Geometry check sheet. Reference: drawing and pictorial views, mm from the part's lowest x, y, z. A direction names the side the tool comes from. Give positions to 0.01 mm unless a question says otherwise; leave off trailing zeros. Write each loop counter-clockwise with the first axis right and the second up, starting at its lowest first coordinate (ties: lowest second). Pieces come first, ordered by that corner, then holes. Notation, with made-up numbers: (64.5, 33.25) - (97.5, 33.25) arc R18 ccw to (97.5, 55.25) - close; hole circle Ø6 at (-9, 28). An arc over 180 degrees is marked (long way). Write item = value, one per line. Start each with the question number.
(1) Section check A-A, the plane x = 3. Enter the section's corners in (y, z), plus the area to 3 significant figures.
(2) Access from +Z, -Z, +X, -X, +Y, -Y to the whole of each face (thin tool, end or side, straight path). Record for the marked faces 1 and 2.
(3) Section check D-D, the plane x = 16.5. Enter the section's corners in (y, z), plus the area to 3 significant figures.
(4) Section check B-B, the plane z = 5.5. Enter the section's corners in (x, y), plus the area to 3 significant figures.
(5) Thickness scan on L1, parallel to Z at x = 6, y = 21; L2, parallel to X at y = 13.5, z = 5; L3, parallel to X at y = 4.75, z = 1.5. Record the ranges inside material, lowest first.
(6) Section check C-C, the plane y = 5. Enter the section's corners in (x, z), plus the area to 3 significant figures.
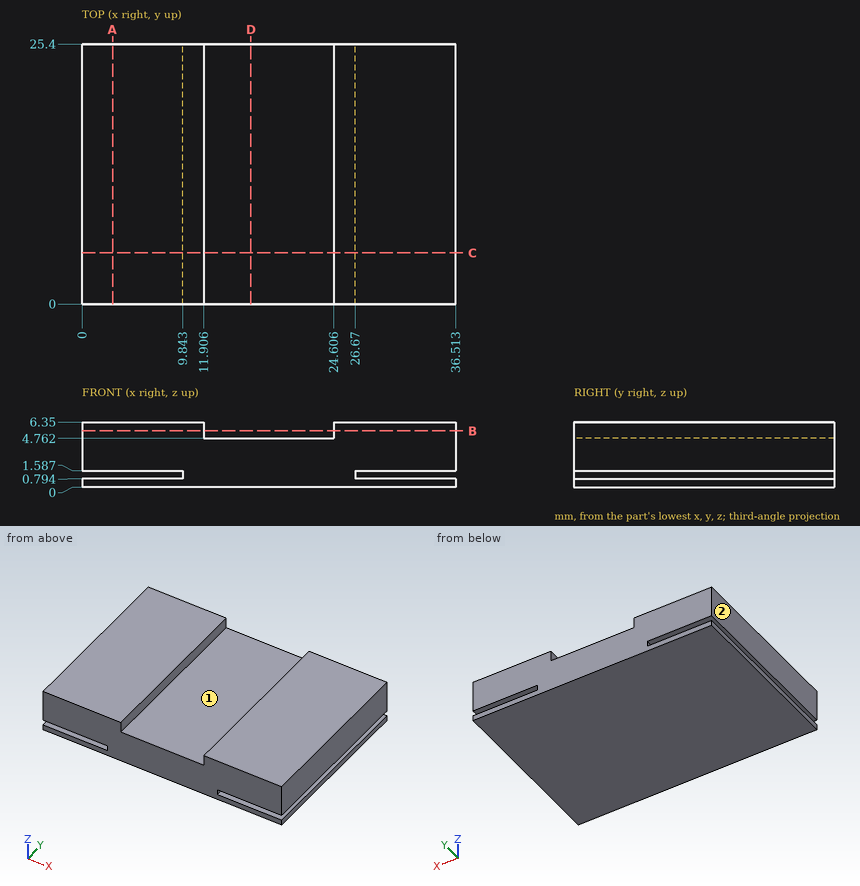
Model answer:
q1.outline = (0, 0) - (25.4, 0) - (25.4, 0.79) - (0, 0.79) - close; (0, 1.59) - (25.4, 1.59) - (25.4, 6.35) - (0, 6.35) - close
q1.area = 141 mm²
q2.face_1 = +Z, +Y, -Y
q2.face_2 = +Z, -Z, -X, +Y, -Y
q3.outline = (0, 0) - (25.4, 0) - (25.4, 4.76) - (0, 4.76) - close
q3.area = 121 mm²
q4.outline = (0, 0) - (11.91, 0) - (11.91, 25.4) - (0, 25.4) - close; (24.61, 0) - (36.51, 0) - (36.51, 25.4) - (24.61, 25.4) - close
q4.area = 605 mm²
q5.L1 = 0 to 0.79, 1.59 to 6.35
q5.L2 = 0 to 11.91, 24.61 to 36.51
q5.L3 = 9.84 to 26.67
q6.outline = (0, 0) - (36.51, 0) - (36.51, 0.79) - (26.67, 0.79) - (26.67, 1.59) - (36.51, 1.59) - (36.51, 6.35) - (24.61, 6.35) - (24.61, 4.76) - (11.91, 4.76) - (11.91, 6.35) - (0, 6.35) - (0, 1.59) - (9.84, 1.59) - (9.84, 0.79) - (0, 0.79) - close
q6.area = 196 mm²
